```python
from build123d import *

# Parameters (mm, degrees)
F0_W      = 152.4
F0_H      = 19.05
F0_R      = 6.35
F1_DEPTH  = 19.05
F2_R      = 6.35
F3_DEPTH  = 25.4
F4_R      = 3.5000057
F5_DEPTH  = 25.4
F6_R      = 3.5000057
F7_DEPTH  = 22.86
F8_W      = 1.27
F8_H      = 19.05
F9_DEPTH  = 25.4
F11_DEPTH = 25.4
F13_DEPTH = 25.4
F15_DEPTH = 25.4
F17_DEPTH = 7.62
F18_DEPTH = 1.27


with BuildPart() as f1:
    # F0 (on Top) → F1 (new body)
    with BuildSketch(Plane.XY):
        with Locations((-5.8522596955, 7.7582320684)):
            Rectangle(F0_W, F0_H)
        with Locations((-37.6022596955, 7.7582320684)):
            Circle(F0_R, mode=Mode.SUBTRACT)
        with Locations((-7.1222596955, 7.7582320684)):
            Circle(F0_R, mode=Mode.SUBTRACT)
        with Locations((23.3577403045, 7.7582320684)):
            Circle(F0_R, mode=Mode.SUBTRACT)
    extrude(amount=F1_DEPTH)

    # F2 (on face) → F3 (cut)
    with BuildSketch(Plane(origin=(0, 17.2832320684, 0), x_dir=(-1, 0, 0), z_dir=(0, 1, 0))):
        with Locations((21.8949988484, 9.525)):
            Circle(F2_R)
        with Locations((-39.0761239581, 9.525)):
            Circle(F2_R)
        with Locations((-8.5961239581, 9.525)):
            Circle(F2_R)
    extrude(amount=-F3_DEPTH, mode=Mode.SUBTRACT)

    # F4 (on face) → F5 (cut)
    with BuildSketch(Plane(origin=(-82.0522596955, 0, 0), x_dir=(0, -1, 0), z_dir=(-1, 0, 0))):
        with Locations((-7.7582320684, 9.525)):
            Circle(F4_R)
    extrude(amount=-F5_DEPTH, mode=Mode.SUBTRACT)

    # F6 (on face) → F7 (cut)
    with BuildSketch(Plane.YZ.offset(70.3477403045)):
        with Locations((7.7582320684, 9.525)):
            Circle(F6_R)
    extrude(amount=-F7_DEPTH, mode=Mode.SUBTRACT)

    # F8 (on face) → F9 (join)
    with BuildSketch(Plane.XY.offset(19.05)):
        with Locations((-81.4172596955, 7.7582320684)):
            Rectangle(F8_W, F8_H)
    extrude(amount=F9_DEPTH)

    # F10 (on face) → F11 (join)
    with BuildSketch(Plane(origin=(0, 17.2832320684, 0), x_dir=(-1, 0, 0), z_dir=(0, 1, 0))):
        Polygon((80.7822596955, 44.45), (80.7822596955, 19.05), (80.7822596955, 0), (82.0522596955, 0), (82.0522596955, 44.45), align=None)
    extrude(amount=F11_DEPTH)

    # F12 (on face) → F13 (join)
    with BuildSketch(Plane.XZ.offset(1.7667679316)):
        Polygon((-80.7822596955, 0), (-80.7822596955, 19.05), (-80.7822596955, 44.45), (-82.0522596955, 44.45), (-82.0522596955, 0), align=None)
    extrude(amount=F13_DEPTH)

    # F14 (on face) → F15 (join)
    with BuildSketch(Plane(origin=(0, 0, 0), x_dir=(1, 0, 0), z_dir=(0, 0, -1))):
        Polygon((-80.7822596955, -17.2832320684), (-80.7822596955, 1.7667679316), (-80.7822596955, 27.1667679316), (-82.0522596955, 27.1667679316), (-82.0522596955, -42.6832320684), (-80.7822596955, -42.6832320684), align=None)
    extrude(amount=F15_DEPTH)

    # F16 (on face) → F17 (cut)
    with BuildSketch(Plane.XZ.offset(1.7667679316)):
        with BuildLine():
            Line((58.9223379939, 9.525), (61.7163379939, 9.525))
            ThreePointArc((61.7163379939, 9.525), (60.3193379939, 10.922), (58.9223379939, 9.525))
        make_face()
        with BuildLine():
            ThreePointArc((58.9223379939, 9.525), (60.3193379939, 8.128), (61.7163379939, 9.525))
            Line((61.7163379939, 9.525), (58.9223379939, 9.525))
        make_face()
    extrude(amount=-F17_DEPTH, mode=Mode.SUBTRACT)

    # F16 (on face) → F18 (cut)
    with BuildSketch(Plane.XZ.offset(1.7667679316)):
        with BuildLine():
            ThreePointArc((57.6650379939, 9.525), (60.3193379939, 6.8707), (62.9736379939, 9.525))
            Line((62.9736379939, 9.525), (61.7163379939, 9.525))
            ThreePointArc((61.7163379939, 9.525), (60.3193379939, 8.128), (58.9223379939, 9.525))
            Line((58.9223379939, 9.525), (57.6650379939, 9.525))
        make_face()
        with BuildLine():
            Line((61.7163379939, 9.525), (62.9736379939, 9.525))
            ThreePointArc((62.9736379939, 9.525), (60.3193379939, 12.1793), (57.6650379939, 9.525))
            Line((57.6650379939, 9.525), (58.9223379939, 9.525))
            ThreePointArc((58.9223379939, 9.525), (60.3193379939, 10.922), (61.7163379939, 9.525))
        make_face()
    extrude(amount=-F18_DEPTH, mode=Mode.SUBTRACT)


solid = f1.part
```
Verification items for the finished model (mm, model axes). A direction names the side the tool comes from. Coordinates: 2 decimals unless noted, no trailing zeros. Loops run counter-clockwise (first coordinate to the right, second up) from the corner with the lowest first, then second, coordinate; pieces in that order, holes last. Notation, with made-up numbers: (30, 32) -> (59, 32) arc R11 cw to (59, 46) -> close; hole circle Ø6 at (28.25, -12). An arc over 180 degrees is marked (long way). Put each result on its own line as item: value.
1. Section check A-A, the plane y = 28. Record the boundary of the cut face in (x, z), then the cut area to 3 significant figures.
Result set:
outline: (-82.05, -25.4) -> (-80.78, -25.4) -> (-80.78, 44.45) -> (-82.05, 44.45) -> close
area: 88.7 mm^2
2. Section check B-B, the plane z = 36. Record the boundary of the cut face in (x, y).
Result set:
outline: (-82.05, -27.17) -> (-80.78, -27.17) -> (-80.78, 42.68) -> (-82.05, 42.68) -> close
3. Section check C-C, the plane x = 53. Record the boundary of the cut face in (y, z) (3 decimals), then the cut area to 3 significant figures.
Result set:
outline: (-1.767, 0) -> (17.283, 0) -> (17.283, 19.05) -> (-1.767, 19.05) -> close; hole circle Ø7 at (7.758, 9.525)
area: 324 mm^2
4. Tool access check on faces 4 (the face through (-56.652, 8, 10)), 5 (the face through (-6, 17.283, 9)), 6 (the face through (61.715, 1.991, 9.464)). Record the directions out of +Z, -Z, +X, -X, +Y, -Y that give a thin tool (end or side, any length) a straight path to the whole face; none if there is none.
Result set:
face 4: -X
face 5: +Z, -Z, +X, +Y
face 6: -Y
5. Gauge pin test, flat ends, axial feed: P1, Ø1.6, axis at x = 60.5, z = 10, coming from the -Y side; P2, Ø12, axis at x = 36, y = -6, coming from the -Z side; P3, Ø6.5, axis at y = 7.76, z = 9.52, coming from the -X side. Record the tip position at first contact, or that the pin passes through.
Result set:
P1: stops at y = 11.02
P2: stops at z = 0
P3: stops at x = -56.65
6. Thickness scan on line 1 (X direction, y = 8, z = 3); line 2 (Y direction, x = 61, z = 16); line 3 (X direction, y = 3.5, z = 28). Record the ranges inside material, lowest first.
Result set:
line 1: x = -82.05 to -43.95, -31.26 to -13.47, -0.78 to 17.01, 29.7 to 70.35
line 2: y = -1.77 to 17.28
line 3: x = -82.05 to -80.78
7. Mould release check, pull along Z, two halves, no side actions. Record for faces 1 (the face through (70.348, 8, 14)), 2 (the face through (62.77, -1.14, 8.51)), 3 (the face through (-6.28, 14.24, 0)): pulls with the +Z half, pulls with the -Z half, needs draft (parallel to the pull), parting line crosses it, or undercut.
Result set:
face 1: needs draft
face 2: undercut
face 3: pulls with the -Z half
